Model file for the job. Use its own axes, mm. A direction names the side the tool comes from. Coordinates: 2 decimals unless noted, no trailing zeros. Write each loop counter-clockwise with the first axis right and the second up, starting at its lowest first coordinate (ties: lowest second). Pieces come first, ordered by that corner, then holes. Notation, with made-up numbers: M -28,89.5 L -13,89.5 A31 cw -13,113.5 Z; hole C 18.5,56.25 d2. An arc over 180 degrees is marked long. Put each result on its own line as item: value. Start each with the question number.
Q1. Pull direction Y, two halves, no side cores. Call faces 1 (the flat face through (0, 195, 0)), 2 (the cylindrical face through (-35.916, 1.644, 3.042)), 3 (the cylindrical face through (-1.04, 257.79, 3.04)): pulls with the +Y half, pulls with the -Y half, needs draft (parallel to the pull), parting line crosses it, or undercut.
Q2. Cut at B-B (x = -19). Write the cut outline in (y, z), then the cut area to 3 significant figures.
Q3. Cut at A-A (z = 1.2). Write the cut outline in (x, y), then the cut area to 3 significant figures.
Q4. Drop flat-ended pins along their axis: pin 1 (9.5 mm diameter, centred on x = 0, y = 249.87, fed in from +Z); pin 2 (1 mm diameter, centred on y = 107, z = 4.5, fed in from -X); pin 3 (3 mm diameter, centred on y = 191.5, z = 1.5, fed in from +X); pin 4 (1 mm diameter, centred on y = 211.5, z = 3, fed in from +X). Give the stop position or say it passes through.
Q5. Drill centre lines: line 1 along X through (y, z) = (249.5, 3.2); line 2 along X through (y, z) = (124, 5.5); line 3 along Y through (x, z) = (25, 1.45). Where is each one in solid material? Low to high.
Q6. Cut at C-C (y = 58). Write the cut outline in (x, z), then the cut area to 3 significant figures.
Q7. Which spindle directions (+Z, -Z, +X, -X, +Y, -Y) get a long thin tool onto all of the face, cutting with end or side? Do faces 4 (the flat face through (-29.249, 125, 3)), 5 (the cylindrical face through (-31.88, 314.08, 3.04)), 6 (the flat face through (-52.255, 247.136, 2.958)). Say none if no direction does.
Q8. Cut at D-D (x = 15). Write the cut outline in (y, z), then the cut area to 3 significant figures.
```python
from build123d import *

# Parameters (mm, degrees)
F1_DEPTH = 6
F2_R     = 7.9883
F3_DEPTH = 25.4
F6_DEPTH = 25.4
F7_R     = 6.35


with BuildPart() as f1:
    # F0 (on Top) → F1 (new body)
    with BuildSketch(Plane.XY):
        with BuildLine():
            Line((1.470284, 287.84881), (0, 0))
            Line((0, 0), (36.98494, 0))
            Line((36.98494, 0), (58.59907, 80.73898))
            Line((58.59907, 80.73898), (58.59907, 182.05958))
            Line((58.59907, 182.05958), (50.6857, 315.67628))
            Line((50.6857, 315.67628), (34.044278, 314.690702))
            ThreePointArc((34.044278, 314.690702), (22.258545, 295.807244), (1.470284, 287.84881))
        make_face()
        with BuildLine():
            Line((-36.98301, 0.377816), (0, 0))
            Line((0, 0), (1.470284, 287.84881))
            ThreePointArc((1.470284, 287.84881), (-19.235594, 296.019189), (-30.82781, 315.022057))
            Line((-30.82781, 315.022057), (-47.458296, 316.177583))
            Line((-47.458296, 316.177583), (-56.736201, 182.648693))
            Line((-56.736201, 182.648693), (-57.771231, 81.33338))
            Line((-57.771231, 81.33338), (-36.98301, 0.377816))
        make_face()
    extrude(amount=F1_DEPTH)

    # F2 (on face) → F3 (cut)
    with BuildSketch(Plane.XY.offset(6)):
        with Locations((0, 249.86996)):
            Circle(F2_R)
        with Locations((0, 26.06802)):
            Circle(F2_R)
    extrude(amount=-F3_DEPTH, mode=Mode.SUBTRACT)

    # F5 (on face) → F6 (cut)
    with BuildSketch(Plane.XY.offset(6)):
        with BuildLine():
            ThreePointArc((-29.24937, 96.96323), (-20.682428, 76.280802), (0, 67.71386))
            ThreePointArc((0, 67.71386), (20.682428, 76.280802), (29.24937, 96.96323))
            Line((29.24937, 96.96323), (29.24937, 152.81021))
            ThreePointArc((29.24937, 152.81021), (20.682428, 173.492638), (0, 182.05958))
            ThreePointArc((0, 182.05958), (-20.682428, 173.492638), (-29.24937, 152.81021))
            Line((-29.24937, 152.81021), (-29.24937, 96.96323))
        make_face()
    extrude(amount=-F6_DEPTH, mode=Mode.SUBTRACT)

    # F7
    f7_edges = [f1.edges().sort_by_distance(p)[0] for p in [
        (-36.98301, 0.377816, 3),
        (36.98494, 0, 3),
        (50.6857, 315.67628, 3),
        (34.044278, 314.690702, 3),
        (-30.82781, 315.022057, 3),
        (-47.458296, 316.177583, 3),
    ]]
    fillet(f7_edges, radius=F7_R)


solid = f1.part
```
Computed values:
1. face 1: needs draft
1. face 2: pulls with the -Y half
1. face 3: undercut
2. outline: M 0.19,0 L 74.73,0 L 74.73,6 L 0.19,6 Z; M 175.05,0 L 295.82,0 L 295.82,6 L 175.05,6 Z
2. area: 1,170 mm2
3. outline: M -57.77,81.33 L -38.2,5.1 A6.35 ccw -32.11,0.33 L 0,0 L 32.11,0 A6.35 ccw 38.25,4.71 L 58.6,80.74 L 58.6,182.06 L 51.06,309.34 A6.35 ccw 44.35,315.3 L 38.46,314.95 A6.35 ccw 32.87,310.79 A35 cw 1.47,287.85 A35 cw -29.69,311.11 A6.35 ccw -35.24,315.33 L -41.12,315.74 A6.35 ccw -47.9,309.84 L -56.74,182.65 Z; hole M -29.25,96.96 A29.25 ccw 29.25,96.96 L 29.25,152.81 A29.25 ccw -29.25,152.81 Z; hole C 0,26.07 d15.98; hole C 0,249.87 d15.98
3. area: 25,900 mm2
4. pin 1: through
4. pin 2: x = -57.51
4. pin 3: x = 58.13
4. pin 4: x = 56.89
5. line 1: -52.09 to -7.98, 7.98 to 54.6
5. line 2: -57.34 to -29.25, 29.25 to 58.6
5. line 3: 0 to 81.78, 167.99 to 298.32
6. outline: M -51.78,0 L 52.51,0 L 52.51,6 L -51.78,6 Z
6. area: 626 mm2
7. face 4: +Z, -Z
7. face 5: +Z, -Z, +Y
7. face 6: +Z, -Z, -X, +Y
8. outline: M 0,0 L 71.85,0 L 71.85,6 L 0,6 Z; M 177.92,0 L 291.2,0 L 291.2,6 L 177.92,6 Z
8. area: 1,110 mm2
